Geometry check sheet. Reference: the model listing, model coordinates, mm. Face numbers are marked on the shaded views. A direction names the side the tool comes from. Round coordinates to 2 decimals unless told otherwise and drop trailing zeros. Loops run counter-clockwise (first coordinate to the right, second up) from the corner with the lowest first, then second, coordinate; pieces in that order, holes last. Notation, with made-up numbers: (20, -38) - (24, -38) arc R21 cw to (24, -19) - close; hole circle Ø10 at (9.5, 89). An arc over 180 degrees is marked (long way). Answer in a Markdown table with one row per item. Add a question column.
```python
from build123d import *

# Parameters (mm, degrees)
F0_R     = 19.685
F1_DEPTH = 16.764
F2_R     = 10.212252
F3_DEPTH = 13.97
F4_R     = 3.175
F5_DEPTH = 12.192


with BuildPart() as f1:
    # F0 (on Front) → F1 (new body)
    with BuildSketch(Plane.XZ):
        Circle(F0_R)
    extrude(amount=F1_DEPTH)

    # F2 (on face) → F3 (cut)
    with BuildSketch(Plane.XZ.offset(16.764)):
        Circle(F2_R)
    extrude(amount=-F3_DEPTH, mode=Mode.SUBTRACT)

    # F4 (on face) → F5 (join)
    with BuildSketch(Plane(origin=(0, 0, 0), x_dir=(-1, 0, 0), z_dir=(0, 1, 0))):
        Circle(F4_R)
    extrude(amount=F5_DEPTH)


solid = f1.part
```
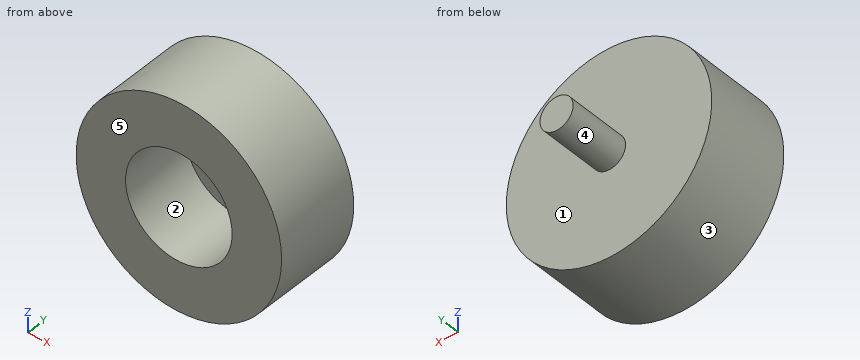
Q1. Depth check by flat-ended pin: P1, Ø12, axis at x = -1, y = 5.5, coming from the +Z side (3 decimals); P2, Ø2, axis at x = 1.5, y = -11, coming from the -Z side; P3, Ø8, axis at x = 5.5, z = -1, coming from the -Y side. Enter the tip coordinate at first touch or a pass-through.
Q2. Cross-section at C-C, the plane y = -5.25. Enter the section's corners in (x, z) (1 decimal).
Q3. Cross-section at A-A, the plane z = 0. Enter the section's corners in (x, y) (3 decimals), plus the area to 3 significant figures.
Q4. Cross-section at B-B, the plane x = 0. Enter the section's corners in (y, z) (3 decimals).
Q5. Cross-section at D-D, the plane y = 5. Enter the section's corners in (x, z) (3 decimals), plus the area to 3 significant figures.
Q6. Set-up check for the marked faces 4 and 5: record each of +Z, -Z, +X, -X, +Y, -Y from which the full face is reachable in a straight line by a thin tool's end or side.
Q7. Scan lines: line 1 (Z direction, x = 0, y = -5.25) (3 decimals); line 2 (Y direction, x = 10, z = 11); line 3 (X direction, y = -5.5, z = 9). Record each from-to range of solid material in increasing order. Write a range as from..to.
Q8. Release check for a two-part mould opening along Z. For the marked faces 1, 2 and 3 record: +Z half, -Z half, draft (parallel to the pull), parting line (faces both ways), or undercut.
Check sheet entries:
| question | item | result |
|---|---|---|
| 1 | P1 | z = 19.685 |
| 1 | P2 | z = -19.68 |
| 1 | P3 | y = -2.79 |
| 2 | outline | circle Ø39.4 at (0, 0); hole circle Ø20.4 at (0, 0) |
| 3 | outline | (-19.685, -16.764) - (-10.212, -16.764) - (-10.212, -2.794) - (10.212, -2.794) - (10.212, -16.764) - (19.685, -16.764) - (19.685, 0) - (3.175, 0) - (3.175, 12.192) - (-3.175, 12.192) - (-3.175, 0) - (-19.685, 0) - close |
| 3 | area | 452 mm² |
| 4 | outline | (-16.764, -19.685) - (0, -19.685) - (0, -3.175) - (12.192, -3.175) - (12.192, 3.175) - (0, 3.175) - (0, 19.685) - (-16.764, 19.685) - (-16.764, 10.212) - (-2.794, 10.212) - (-2.794, -10.212) - (-16.764, -10.212) - close |
| 5 | outline | circle Ø6.35 at (0, 0) |
| 5 | area | 31.7 mm² |
| 6 | face 4 | +Y |
| 6 | face 5 | +Z, -Z, +X, -X, -Y |
| 7 | line 1 | -19.685..-10.212, 10.212..19.685 |
| 7 | line 2 | -16.76..0 |
| 7 | line 3 | -17.51..-4.83, 4.83..17.51 |
| 8 | face 1 | draft |
| 8 | face 2 | undercut |
| 8 | face 3 | parting line |
